CAD build for the part. Positions are in the model's coordinates, mm. Face numbers are marked on the shaded views. A direction names the side the tool comes from. Coordinates: 2 decimals unless noted, no trailing zeros. Loops run counter-clockwise (first coordinate to the right, second up) from the corner with the lowest first, then second, coordinate; pieces in that order, holes last. Notation, with made-up numbers: (86.25, 79) -> (91.25, 79) arc R19 cw to (91.25, 108) -> close; hole circle Ø6 at (1, -11.5). An arc over 180 degrees is marked (long way). Return JSON: item names as keys, results as strings. Group by question number.
(1) Saw through at A-A on y = 34. Write the cut outline in (x, z), then the cut area to 3 significant figures.
(2) Probe L1, parallel to Y at x = 0, z = 50.7; L2, parallel to Y at x = 51.9, z = 0; L3, parallel to Z at x = 17.5, y = 23. List the from-to ranges inside material, lowest first.
(3) Saw through at C-C on x = 26.5. Write the cut outline in (y, z).
(4) Mould opens along Z. For the marked faces 1, 2, 3 and 4 say: pulls with the +Z half, pulls with the -Z half, needs draft (parallel to the pull), parting line crosses it, or undercut.
(5) Saw through at D-D on z = -5. Write the cut outline in (x, y), then the cut area to 3 significant figures.
(6) Saw through at B-B on z = -19.5. Write the cut outline in (x, y), then the cut area to 3 significant figures.
(7) Flat gauge pins, fed straight in: pin 1 Ø2.5 at (y, z) = (-7.5, -51.5) entering from +X; pin 2 Ø3 at (x, z) = (-0.5, 4.5) entering from -Y; pin 3 Ø0.9 at (y, z) = (-9.5, -50.5) entering from -X. Where does each tip first touch, or does it go through?
(8) Tool access for the marked faces 5, 6 and 7: list every direction of +Z, -Z, +X, -X, +Y, -Y with a clear straight run to the whole face (end or side of a thin tool).
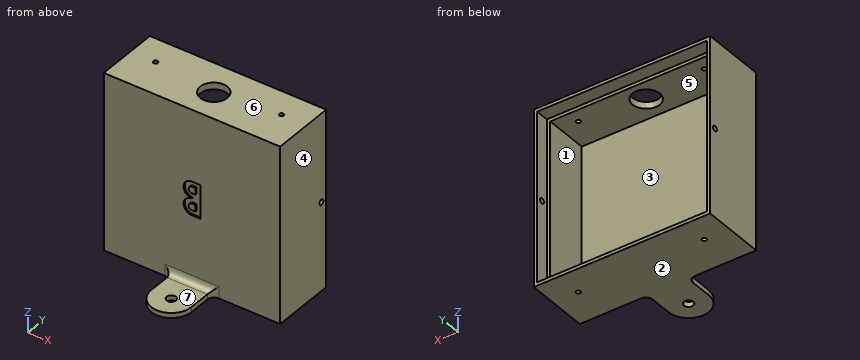
```python
from build123d import *

# Parameters (mm, degrees)
SKETCH1_W           = 105
SKETCH1_H           = 105
BOSS_EXTRUDE1_DEPTH = 38
SKETCH2_W           = 97
SKETCH2_H           = 97
CUT_EXTRUDE1_DEPTH  = 34
SKETCH3_W           = 101
SKETCH3_H           = 101
CUT_EXTRUDE2_DEPTH  = 8
SKETCH5_R           = 1.6
CUT_EXTRUDE3_DEPTH  = 106
SKETCH6_R           = 2.75
BOSS_EXTRUDE2_DEPTH = 3
FILLET1_R           = 4
CUT_EXTRUDE4_REACH  = 6
SKETCH7_R           = 8.1
CUT_EXTRUDE5_DEPTH  = 1
SKETCH11_R          = 1.3
CUT_EXTRUDE6_DEPTH  = 106


with BuildPart() as part:
    # Sketch1 → Boss-Extrude1 (new body)
    with BuildSketch(Plane(origin=(0, 0, 0), x_dir=(1, 0, 0), z_dir=(0, 1, 0))):
        Rectangle(SKETCH1_W, SKETCH1_H)
    extrude(amount=BOSS_EXTRUDE1_DEPTH)

    # Sketch2 → Cut-Extrude1 (cut)
    with BuildSketch(Plane(origin=(0, 38, 0), x_dir=(1, 0, 0), z_dir=(0, 1, 0))):
        Rectangle(SKETCH2_W, SKETCH2_H)
    extrude(amount=-CUT_EXTRUDE1_DEPTH, mode=Mode.SUBTRACT)

    # Sketch3 → Cut-Extrude2 (cut)
    with BuildSketch(Plane(origin=(0, 38, 0), x_dir=(1, 0, 0), z_dir=(0, 1, 0))):
        Rectangle(SKETCH3_W, SKETCH3_H)
    extrude(amount=-CUT_EXTRUDE2_DEPTH, mode=Mode.SUBTRACT)

    # Sketch5 → Cut-Extrude3 (cut, through all)
    with BuildSketch(Plane(origin=(52.5, 0, 0), x_dir=(0, 0, -1), z_dir=(1, 0, 0))):
        with Locations((0, 34)):
            Circle(SKETCH5_R)
    extrude(amount=-CUT_EXTRUDE3_DEPTH, mode=Mode.SUBTRACT)

    # Sketch6 → Boss-Extrude2 (add)
    with BuildSketch(Plane(origin=(0, 0, -52.5), x_dir=(-1, 0, 0), z_dir=(0, 0, -1))):
        with BuildLine():
            Line((-12, 0), (12, 0))
            Line((12, 0), (12, -5))
            Line((12, -5), (12, -17))
            ThreePointArc((12, -17), (0, -29), (-12, -17))
            Line((-12, -17), (-12, -5))
            Line((-12, -5), (-12, 0))
        make_face()
        with Locations((0, -17)):
            Circle(SKETCH6_R, mode=Mode.SUBTRACT)
    extrude(amount=-BOSS_EXTRUDE2_DEPTH)

    # Fillet1
    fillet1_edges = [part.edges().sort_by_distance(p)[0] for p in [
        (0, 0, -49.5),
        (12, 0, -51),
        (-12, 0, -51),
    ]]
    fillet(fillet1_edges, radius=FILLET1_R)

    # Sketch7 → Cut-Extrude4 (cut, up to next)
    with BuildSketch(Plane(origin=(0, 0, 48.5), x_dir=(-1, 0, 0), z_dir=(0, 0, -1)), mode=Mode.PRIVATE) as cut_extrude4_sk1:
        with Locations((0, 18)):
            Circle(SKETCH7_R)
    cut_extrude4_tool1 = extrude(cut_extrude4_sk1.sketch, amount=-CUT_EXTRUDE4_REACH, mode=Mode.PRIVATE) & part.part
    add(cut_extrude4_tool1.solids().sort_by_distance((0, 18, 48.5))[0], mode=Mode.SUBTRACT)

    # Sketch10 → Cut-Extrude5 (cut)
    with BuildSketch(Plane.XZ):
        with BuildLine():
            Line((5, -10), (0, -10))
            ThreePointArc((0, -10), (-5, -5), (0, 0))
            ThreePointArc((0, 0), (-5, 5), (0, 10))
            Line((0, 10), (5, 10))
            Line((5, 10), (5, -10))
        make_face()
        with BuildLine():
            Line((0, -7), (2, -7))
            Line((2, -7), (2, -3))
            Line((2, -3), (0, -3))
            ThreePointArc((0, -3), (-2, -5), (0, -7))
        make_face(mode=Mode.SUBTRACT)
        with BuildLine():
            Line((0, 3), (2, 3))
            Line((2, 3), (2, 7))
            Line((2, 7), (0, 7))
            ThreePointArc((0, 7), (-2, 5), (0, 3))
        make_face(mode=Mode.SUBTRACT)
    extrude(amount=-CUT_EXTRUDE5_DEPTH, mode=Mode.SUBTRACT)

    # Sketch11 → Cut-Extrude6 (cut, through all)
    with BuildSketch(Plane.XY.offset(52.5)):
        with Locations((-37.5, 22)):
            Circle(SKETCH11_R)
        with Locations((37.5, 22)):
            Circle(SKETCH11_R)
    extrude(amount=-CUT_EXTRUDE6_DEPTH, mode=Mode.SUBTRACT)


solid = part.part
```
Geometry results:
{
 "1": {"outline": "(-52.5, -52.5) -> (52.5, -52.5) -> (52.5, -1.6) -> (50.5, -1.6) -> (50.5, -50.5) -> (-50.5, -50.5) -> (-50.5, -1.6) -> (-52.5, -1.6) -> close; (-52.5, 1.6) -> (-50.5, 1.6) -> (-50.5, 50.5) -> (50.5, 50.5) -> (50.5, 1.6) -> (52.5, 1.6) -> (52.5, 52.5) -> (-52.5, 52.5) -> close", "area": "811 mm²"},
 "2": {"L1": "0 to 9.9, 26.1 to 38", "L2": "0 to 32.4, 35.6 to 38", "L3": "-52.5 to -48.5, 48.5 to 52.5"},
 "3": {"outline": "(0, -52.5) -> (38, -52.5) -> (38, -50.5) -> (30, -50.5) -> (30, -48.5) -> (4, -48.5) -> (4, 48.5) -> (30, 48.5) -> (30, 50.5) -> (38, 50.5) -> (38, 52.5) -> (0, 52.5) -> close"},
 "4": {"face 1": "undercut", "face 2": "pulls with the -Z half", "face 3": "undercut", "face 4": "needs draft"},
 "5": {"outline": "(-52.5, 0) -> (-5, 0) -> (-5, 1) -> (-2, 1) -> (-2, 0) -> (2, 0) -> (2, 1) -> (5, 1) -> (5, 0) -> (52.5, 0) -> (52.5, 38) -> (50.5, 38) -> (50.5, 30) -> (48.5, 30) -> (48.5, 4) -> (-48.5, 4) -> (-48.5, 30) -> (-50.5, 30) -> (-50.5, 38) -> (-52.5, 38) -> close", "area": "654 mm²"},
 "6": {"outline": "(-52.5, 0) -> (52.5, 0) -> (52.5, 38) -> (50.5, 38) -> (50.5, 30) -> (48.5, 30) -> (48.5, 4) -> (-48.5, 4) -> (-48.5, 30) -> (-50.5, 30) -> (-50.5, 38) -> (-52.5, 38) -> close", "area": "660 mm²"},
 "7": {"pin 1": "x = 12", "pin 2": "y = 0", "pin 3": "x = -12"},
 "8": {"face 5": "+Y", "face 6": "+Z, +X, -X, +Y, -Y", "face 7": "+Z, +X, -X, -Y"}
}
